```python
from build123d import *

# Parameters (mm, degrees)
SKETCH1_R      = 5.1435
EXTRUDE1_DEPTH = 3.556
SKETCH2_R      = 3.75
EXTRUDE2_DEPTH = 3.175
EXTRUDE3_DEPTH = 4.007423572
FILLET1_R      = 1.27


with BuildPart() as part:
    # Sketch1 → Extrude1 (new body)
    with BuildSketch(Plane.XY):
        Circle(SKETCH1_R)
    extrude(amount=EXTRUDE1_DEPTH)

    # Sketch2 → Extrude2 (add)
    with BuildSketch(Plane(origin=(0, 0, 0), x_dir=(-1, 0, 0), z_dir=(0, 0, -1))):
        with Locations(Location((0, 0, 0), (0, 0, 180))):
            Circle(SKETCH2_R)
    extrude(amount=EXTRUDE2_DEPTH)

    # Sketch3 → Extrude3 (add)
    with BuildSketch(Plane(origin=(0, 0, -3.175), x_dir=(-1, 0, 0), z_dir=(0, 0, -1))):
        Polygon((-3.189571562, -5.5245), (3.189571562, -5.5245), (6.379143124, 0), (3.189571562, 5.5245), (-3.189571562, 5.5245), (-6.379143124, 0), align=None)
    extrude(amount=EXTRUDE3_DEPTH)

    # Fillet1
    fillet1_edges = [part.edges().sort_by_distance(p)[0] for p in [
        (-5.1435, 0, 3.556),
    ]]
    fillet(fillet1_edges, radius=FILLET1_R)


solid = part.part
```
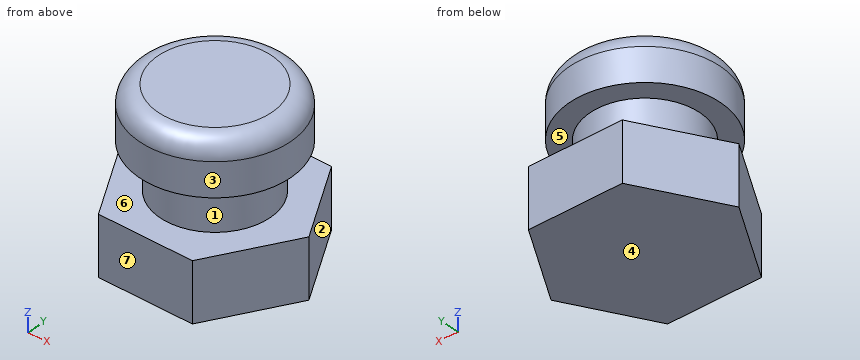
For this review, take the finished solid that the model builds, in its own axes (mm). Face numbers are marked on the shaded views. A direction names the side the tool comes from. Coordinates: 2 decimals unless noted, no trailing zeros. Put each result on its own line as item: value.
1. Machinability: for the marked faces 1, 2 and 3, which of the approach directions +Z, -Z, +X, -X, +Y, -Y give a long, thin tool a straight path to every point of the face, cutting with its end or side? Answer none if there is none.
Values found:
face 1: none
face 2: +Z, -Z, +X, +Y
face 3: +Z
2. Mouldability with a two-part tool opening along Z and no side actions: class the marked faces 4, 5, 6 and 7 as released by +Z, released by -Z, zero draft, split by the parting line, or undercut.
Values found:
face 4: released by -Z
face 5: undercut
face 6: undercut
face 7: zero draft
3. For pin 1 (5 mm diameter, centred on y = 1, z = 2, fed in from -X); pin 2 (1.5 mm diameter, centred on y = -3, z = -1.5, fed in from -X); pin 3 (2 mm diameter, centred on y = -2.5, z = -3, fed in from +X), all flat-tipped, find the tip position at first contact; note any pin that passes through.
Values found:
pin 1: x = -5.14
pin 2: x = -3
pin 3: x = 5.5
4. Wall thickness on probe 1 along Z at (x, y) = (-5.25, 0.25) (3 decimals); probe 2 along X at (y, z) = (3.25, 2.75); probe 3 along Z at (x, y) = (3.75, -1.75) (3 decimals): over which ranges is each line inside the solid? List them lowest first.
Values found:
probe 1: -7.182 to -3.175
probe 2: -3.87 to 3.87
probe 3: -7.182 to -3.175, 0 to 3.528
